Job drawing, mm, ordinate dimensions from the low corner. One solid piece. A direction names the side the tool comes from. Coordinates: 2 decimals unless noted, no trailing zeros. Loops run counter-clockwise (first coordinate to the right, second up) from the corner with the lowest first, then second, coordinate; pieces in that order, holes last. Notation, with made-up numbers: (-2, -19.5) - (33, -19.5) arc R30 cw to (33, 7.5) - close; hole circle Ø8 at (39, 4). An arc over 180 degrees is marked (long way). Use a Markdown table: item, result. Add a question column.
1. Band-saw the part on A-A, the plane y = 0.6. Give the cut face in (x, z).
2. Band-saw the part on B-B, the plane z = 3.75. Give the cut face in (x, y).
3. Drop flat-ended pins along their axis: pin 1 (0.8 mm diameter, centred on x = 11, z = 9, fed in from +Y); pin 2 (3 mm diameter, centred on x = 2, z = 4.5, fed in from +Y); pin 3 (1 mm diameter, centred on x = 4, z = 7, fed in from +Y). Give the stop position or say it passes through.
4. 3-axis set-ups, long thin cutter, end or side, ignore diameter. For the marked faces 1, 2, 3 and 4: which of +Z, -Z, +X, -X, +Y, -Y reach the whole face in a straight line?
5. Band-saw the part on D-D, the plane x = 6.5. Give the cut face in (y, z).
6. Pull direction X, two halves, no side cores. Call the marked faces 5, 6 and 7: pulls with the +X half, pulls with the -X half, needs draft (parallel to the pull), parting line crosses it, or undercut.
7. Band-saw the part on C-C, the plane y = 3.65. Give the cut face in (x, z), plus the area to 3 significant figures.
8. Wall check: probe 1 along X at (y, z) = (0.8, 2.75); probe 2 along X at (y, z) = (2.15, 11.5); probe 3 along Y at (x, z) = (1.5, 2.5). Give the ranges that are in metal, low to high. Write a range as [from, to].
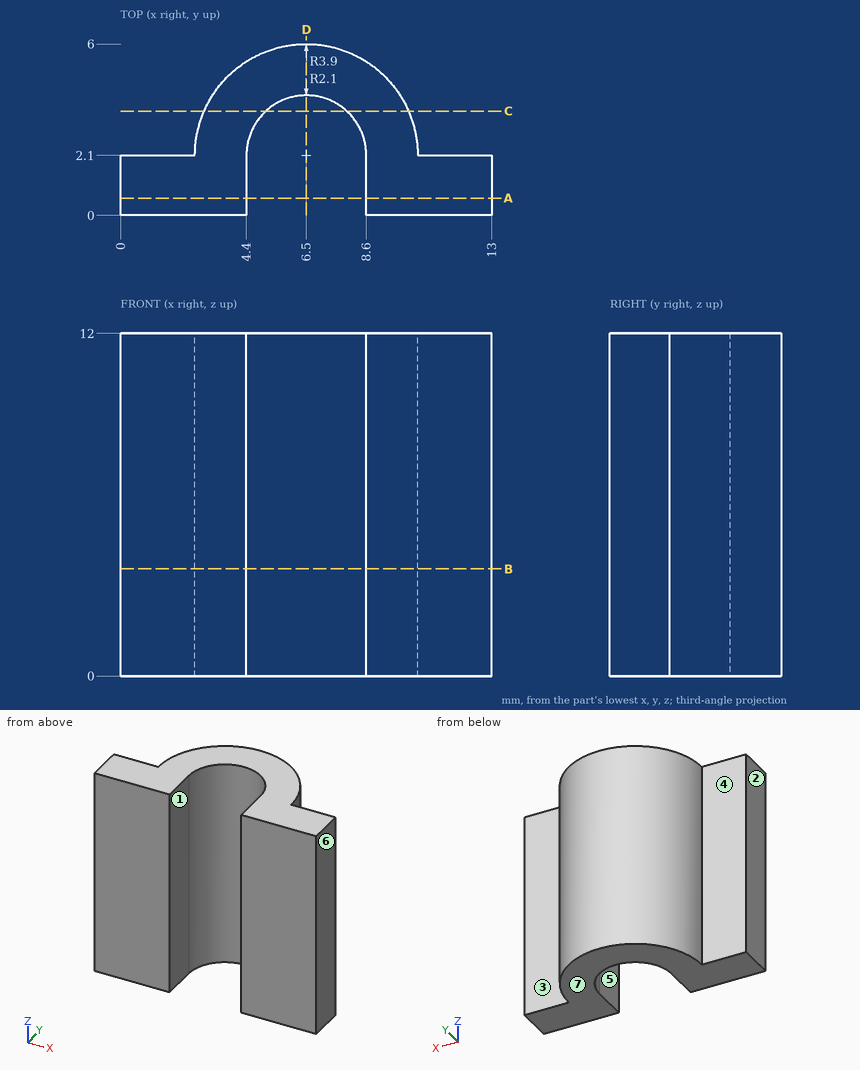
Geometry check:
| question | item | result |
|---|---|---|
| 1 | outline | (0, 0) - (4.4, 0) - (4.4, 12) - (0, 12) - close; (8.6, 0) - (13, 0) - (13, 12) - (8.6, 12) - close |
| 2 | outline | (0, 0) - (4.4, 0) - (4.4, 2.1) arc R2.1 cw to (8.6, 2.1) - (8.6, 0) - (13, 0) - (13, 2.1) - (10.4, 2.1) arc R3.9 ccw to (2.6, 2.1) - (0, 2.1) - close |
| 3 | pin 1 | stops at y = 2.1 |
| 3 | pin 2 | stops at y = 4.59 |
| 3 | pin 3 | stops at y = 5.45 |
| 4 | face 1 | +Z, -Z, -Y |
| 4 | face 2 | +Z, -Z, -X, +Y, -Y |
| 4 | face 3 | +Z, -Z, +X, +Y |
| 4 | face 4 | +Z, -Z, -X, +Y |
| 5 | outline | (4.2, 0) - (6, 0) - (6, 12) - (4.2, 12) - close |
| 6 | face 5 | undercut |
| 6 | face 6 | pulls with the +X half |
| 6 | face 7 | needs draft |
| 7 | outline | (2.92, 0) - (5.08, 0) - (5.08, 12) - (2.92, 12) - close; (7.92, 0) - (10.08, 0) - (10.08, 12) - (7.92, 12) - close |
| 7 | area | 51.9 mm^2 |
| 8 | probe 1 | x = [0, 4.4], [8.6, 13] |
| 8 | probe 2 | x = [2.6, 4.4], [8.6, 10.4] |
| 8 | probe 3 | y = [0, 2.1] |
